from build123d import *

# Parameters (mm, degrees)
F0_W         = 220
F0_H         = 141.9456327772
F1_DEPTH     = 250
F3_W         = 210.672037676
F3_H         = 112.9930540919
F4_DEPTH     = 206
F5_W         = 19.7831674727
F5_H         = 141
F6_DEPTH     = 200
F7_T4_DEPTH  = 275
F7_T10_DEPTH = 275
F7_T16_DEPTH = 275
F7_T23_DEPTH = 275
F7_T29_DEPTH = 275
F8_SIZE      = 5
F9_T1_DEPTH  = 218.5
F10_R        = 5
F11_R        = 5
F12_W        = 90
F12_H        = 50
F13_DEPTH    = 5
F14_W        = 14.7826219899
F14_H        = 8.5
F15_DEPTH    = 3
F16_W        = 14.5
F16_H        = 8.5
F17_DEPTH    = 3


# Not quite as in the source:
# - a fillet or chamfer that OpenCascade refuses, or shapes differently, is made with other operations: its cross-section is extruded or revolved along the edge and cut away or added


with BuildPart() as f1:
    # F0 (on Front) → F1 (new body)
    with BuildSketch(Plane.XZ):
        Rectangle(F0_W, F0_H)
    extrude(amount=F1_DEPTH)

    # F3 (on face) → F4 (cut)
    with BuildSketch(Plane.YZ.offset(110)):
        with Locations((-124.4797622785, -0.6201006472)):
            Rectangle(F3_W, F3_H)
    extrude(amount=-F4_DEPTH, mode=Mode.SUBTRACT)

    # F5 (on face) → F6 (join)
    with BuildSketch(Plane.YZ.offset(110)):
        with Locations((-239.0063405037, -0.1803636551)):
            Rectangle(F5_W, F5_H)
    extrude(amount=F6_DEPTH)

    # F7: fillet of radius 5 on 1 edges, made by hand


with BuildPart() as f7_tool2:
    # F7_s3 → F7_t4 (new body)
    with BuildSketch(Plane.XZ.offset(-12.5)):
        with BuildLine():
            ThreePointArc((105, 70.9728163886), (108.5355339059, 69.5083502945), (110, 65.9728163886))
            Line((110, 65.9728163886), (110, 70.9728163886))
            Line((110, 70.9728163886), (105, 70.9728163886))
        make_face()
    extrude(amount=F7_T4_DEPTH)

    split(bisect_by=Plane.XY.offset(70.3196363449), keep=Keep.TOP)

    split(bisect_by=Plane.XZ.offset(229.1147567674), keep=Keep.BOTTOM)


with BuildPart() as f1_1:
    add(f1.part)

    # F7_t1: cut F7_tool2
    add(f7_tool2.part, mode=Mode.SUBTRACT)


with BuildPart() as f7_tool8:
    # F7_s9 → F7_t10 (new body)
    with BuildSketch(Plane.XZ.offset(-12.5)):
        with BuildLine():
            ThreePointArc((105, 70.9728163886), (108.5355339059, 69.5083502945), (110, 65.9728163886))
            Line((110, 65.9728163886), (110, 70.9728163886))
            Line((110, 70.9728163886), (105, 70.9728163886))
        make_face()
    extrude(amount=F7_T10_DEPTH)

    split(bisect_by=Plane.XY.offset(70.3196363449), keep=Keep.BOTTOM)

    split(bisect_by=Plane.XZ.offset(229.1147567674), keep=Keep.BOTTOM)


with BuildPart() as f1_2:
    add(f1_1.part)

    # F7_t7: cut F7_tool8
    add(f7_tool8.part, mode=Mode.SUBTRACT)


with BuildPart() as f7_tool14:
    # F7_s15 → F7_t16 (new body)
    with BuildSketch(Plane.XZ.offset(-12.5)):
        with BuildLine():
            ThreePointArc((105, 70.9728163886), (108.5355339059, 69.5083502945), (110, 65.9728163886))
            Line((110, 65.9728163886), (110, 70.9728163886))
            Line((110, 70.9728163886), (105, 70.9728163886))
        make_face()
    extrude(amount=F7_T16_DEPTH)

    split(bisect_by=Plane.XZ.offset(248.89792424), keep=Keep.BOTTOM)

    split(bisect_by=Plane.XY.offset(70.3196363449), keep=Keep.TOP)

    split(bisect_by=Plane.XZ.offset(229.1147567674), keep=Keep.TOP)


with BuildPart() as f1_3:
    add(f1_2.part)

    # F7_t13: cut F7_tool14
    add(f7_tool14.part, mode=Mode.SUBTRACT)


with BuildPart() as f7_tool21:
    # F7_s22 → F7_t23 (new body)
    with BuildSketch(Plane.XZ.offset(-12.5)):
        with BuildLine():
            ThreePointArc((105, 70.9728163886), (108.5355339059, 69.5083502945), (110, 65.9728163886))
            Line((110, 65.9728163886), (110, 70.9728163886))
            Line((110, 70.9728163886), (105, 70.9728163886))
        make_face()
    extrude(amount=F7_T23_DEPTH)

    split(bisect_by=Plane.XZ.offset(248.89792424), keep=Keep.TOP)

    split(bisect_by=Plane.XY.offset(70.3196363449), keep=Keep.TOP)


with BuildPart() as f1_4:
    add(f1_3.part)

    # F7_t20: cut F7_tool21
    add(f7_tool21.part, mode=Mode.SUBTRACT)


with BuildPart() as f7_tool27:
    # F7_s28 → F7_t29 (new body)
    with BuildSketch(Plane.XZ.offset(-12.5)):
        with BuildLine():
            ThreePointArc((105, 70.9728163886), (108.5355339059, 69.5083502945), (110, 65.9728163886))
            Line((110, 65.9728163886), (110, 70.9728163886))
            Line((110, 70.9728163886), (105, 70.9728163886))
        make_face()
    extrude(amount=F7_T29_DEPTH)

    split(bisect_by=Plane.XZ.offset(248.89792424), keep=Keep.TOP)

    split(bisect_by=Plane.XY.offset(70.3196363449), keep=Keep.BOTTOM)


with BuildPart() as f1_5:
    add(f1_4.part)

    # F7_t26: cut F7_tool27
    add(f7_tool27.part, mode=Mode.SUBTRACT)

    # F8
    f8_edges = [f1_5.edges().sort_by_distance(p)[0] for p in [
        (208.735431, -229.114757, 70.319636),
    ]]
    chamfer(f8_edges, length=F8_SIZE)

    # F9: fillet of radius 5 on 1 edges, made by hand

    # F9_s2 → F9_t1 (join)
    with BuildSketch(Plane.YZ.offset(-108.5)):
        with BuildLine():
            ThreePointArc((-224.8157811165, -57.1166276932), (-228.3513150224, -55.6521615991), (-229.8157811165, -52.1166276932))
            Line((-229.8157811165, -52.1166276932), (-229.8157811165, -57.1166276932))
            Line((-229.8157811165, -57.1166276932), (-224.8157811165, -57.1166276932))
        make_face()
    extrude(amount=F9_T1_DEPTH)

    # F10
    f10_edges = [f1_5.edges().sort_by_distance(p)[0] for p in [
        (-96, -121.979762, -57.116628),
    ]]
    fillet(f10_edges, radius=F10_R)

    # F11
    f11_edges = [f1_5.edges().sort_by_distance(p)[0] for p in [
        (9.5, -19.143743, -57.116628),
    ]]
    fillet(f11_edges, radius=F11_R)

    # F12 (on face) → F13 (join)
    with BuildSketch(Plane.XZ.offset(248.89792424)):
        with Locations((172.4283844233, 35.1449831093)):
            Rectangle(F12_W, F12_H)
    extrude(amount=F13_DEPTH)

    # F14 (on face) → F15 (join)
    with BuildSketch(Plane.XZ.offset(253.89792424)):
        with Locations((141.7928859591, 48.4116636217)):
            Rectangle(F14_W, F14_H)
    extrude(amount=F15_DEPTH)

    # F16 (on face) → F17 (join)
    with BuildSketch(Plane.XZ.offset(253.89792424)):
        with Locations((166.0626122952, 48.4116636217)):
            Rectangle(F16_W, F16_H)
    extrude(amount=F17_DEPTH)


solid = f1_5.part
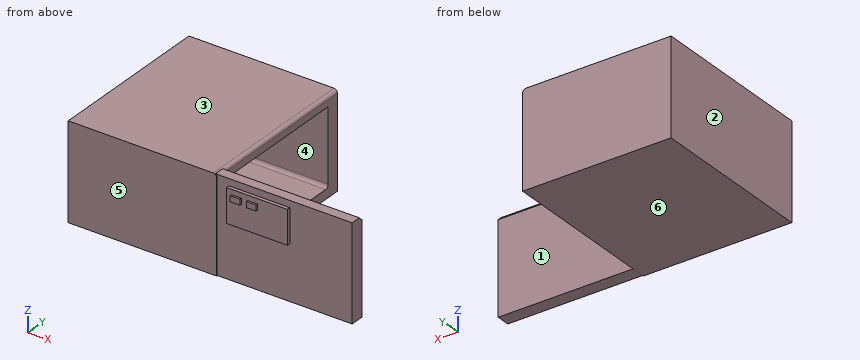
Part model, mm, in its own coordinate system. Face numbers are marked on the shaded views. A direction names the side the tool comes from. Give positions to 0.01 mm unless a question says otherwise; leave off trailing zeros. Loops run counter-clockwise (first coordinate to the right, second up) from the corner with the lowest first, then second, coordinate; pieces in that order, holes last. Notation, with made-up numbers: (75.25, 27.5) -> (133.25, 27.5) arc R18 cw to (133.25, 47.5) -> close; hole circle Ø3 at (-12.75, 88.25). An arc over 180 degrees is marked (long way). Write each question's results on one line, items separated by ' | '. Start each with the question number.
Q1. Band-saw the part on C-C on y = -74. List the corners of the cut face in (x, z).
Q2. Pull direction Z, two halves, no side cores. Call the marked faces 3, 4, 5 and 6: +Z half, -Z half, draft (parallel to the pull), parting line (faces both ways), or undercut.
Q3. Pin check, flat tips, straight feed: P1, Ø5.5, axis at y = -252, z = 32, coming from the +X side; P2, Ø6, axis at x = 183, y = -241.5, coming from the -Z side; P3, Ø3, axis at x = 192.5, z = 34, coming from the +Y side. Stop position of each tip, or through.
Q4. Band-saw the part on D-D on x = 231.5. List the corners of the cut face in (y, z), plus the area to 3 significant figures.
Q5. Which spindle directions (+Z, -Z, +X, -X, +Y, -Y) get a long thin tool onto all of the face, cutting with end or side? Do the marked faces 1 and 2. Say none if no direction does.
Q6. Band-saw the part on A-A on x = -6. List the corners of the cut face in (y, z).
Q7. Band-saw the part on B-B on z = -8.5. List the corners of the cut face in (x, y).
Q8. Wall check: L1, parallel to Y at x = -82.5, z = 50.5; L2, parallel to Z at x = 93, y = -136; L3, parallel to Y at x = 41, z = -63.5. Give the ranges that are in metal, low to high.
Results are:
1) outline: (-110, -70.97) -> (110, -70.97) -> (110, -57.12) -> (-91, -57.12) arc R5 cw to (-96, -52.12) -> (-96, 55.88) -> (110, 55.88) -> (110, 65.97) arc R5 ccw to (105, 70.97) -> (-110, 70.97) -> close
2) face 3: +Z half | face 4: undercut | face 5: draft | face 6: -Z half
3) P1: stops at x = 217.43 | P2: stops at z = -70.68 | P3: stops at y = -229.11
4) outline: (-248.9, -70.68) -> (-229.11, -70.68) -> (-229.11, 65.32) -> (-234.11, 70.32) -> (-248.9, 70.32) -> close | area: 2,780 mm²
5) face 1: +Z, -Z, +X, +Y | face 2: +Z, -Z, -X, +Y, -Y
6) outline: (-250, -70.97) -> (0, -70.97) -> (0, 70.97) -> (-250, 70.97) -> close; hole (-229.82, -52.12) arc R5 ccw to (-224.82, -57.12) -> (-24.14, -57.12) arc R5 ccw to (-19.14, -52.12) -> (-19.14, 55.88) -> (-229.82, 55.88) -> close
7) outline: (-110, -250) -> (110, -250) -> (110, -248.9) -> (310, -248.9) -> (310, -229.11) -> (110, -229.11) -> (110, -229.82) -> (-91, -229.82) arc R5 cw to (-96, -224.82) -> (-96, -24.14) arc R5 cw to (-91, -19.14) -> (110, -19.14) -> (110, 0) -> (-110, 0) -> close
8) L1: y = -250 to -229.82, -19.14 to 0 | L2: z = -70.97 to -57.12, 55.88 to 70.97 | L3: y = -250 to 0
